Answer from the drawing. Dimensions are ordinates in mm from the lowest x, y and z of the part. Round coordinates to 2 decimals unless told otherwise and drop trailing zeros. Order: outer loops, then holes, each group sorted by start corner. A loop starts at its lowest first (then second) coordinate and runs counter-clockwise, first axis right, second up. Notation, with made-up numbers: M 82,74.5 L 126,74.5 A32 cw 126,109.5 Z; hole C 63,-26.75 d6. An arc over 180 degrees is marked long. Write item = value, one per line. Start each with the question number.
(1) A cutting plane is placed at A-A, the plane x = 3.81. Determine the outline of the cut face in (y, z), and give its area (3 significant figures).
(2) A cutting plane is placed at B-B, the plane y = 3.81. Determine the outline of the cut face in (x, z).
(3) Each of these flat-tipped pins is pushed along its axis until it touches: pin 1 (2 mm diameter, centred on x = 18.5, y = 66.5, fed in from -Z); pin 2 (4 mm diameter, centred on x = 3.81, y = 80.264, fed in from +Z); pin 3 (2 mm diameter, centred on x = 82.19, y = 80.264, fed in from -Z). Where does it stop, or does it pass through?
(4) A straight line is drawn through the part: probe 1 along Y at (x, z) = (82.19, 1.6). Find the intervals that lie inside material, in ascending order. Write a range as from..to.
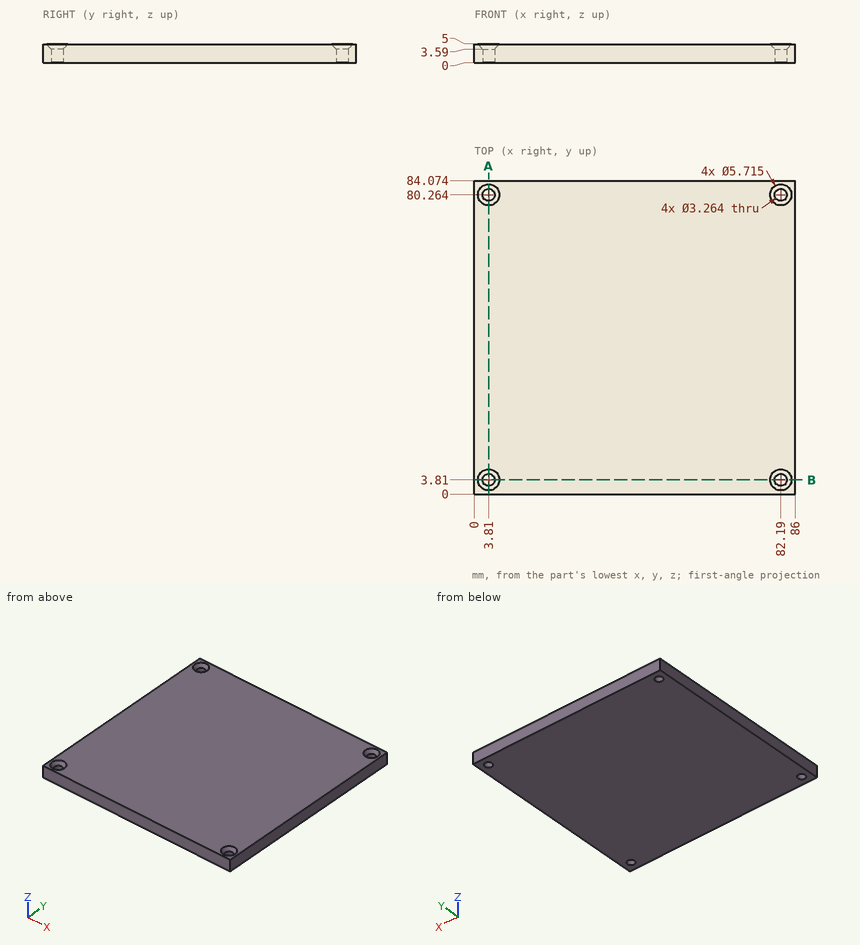
Reported:
q1.outline = M 0,0 L 2.18,0 L 2.18,3.59 L 0.95,5 L 0,5 Z; M 5.44,0 L 78.63,0 L 78.63,3.59 L 77.41,5 L 6.67,5 L 5.44,3.59 Z; M 81.9,0 L 84.07,0 L 84.07,5 L 83.12,5 L 81.9,3.59 Z
q1.area = 384 mm²
q2.outline = M 0,0 L 2.18,0 L 2.18,3.59 L 0.95,5 L 0,5 Z; M 5.44,0 L 80.56,0 L 80.56,3.59 L 79.33,5 L 6.67,5 L 5.44,3.59 Z; M 83.82,0 L 86,0 L 86,5 L 85.05,5 L 83.82,3.59 Z
q3.pin_1 = 0
q3.pin_2 = 4.01
q3.pin_3 = through
q4.probe_1 = 0..2.18, 5.44..78.63, 81.9..84.07
